CAD build for the part. Positions are in the model's coordinates, mm. A direction names the side the tool comes from. Coordinates: 2 decimals unless noted, no trailing zeros. Order: outer loops, then holes, each group sorted by start corner. A loop starts at its lowest first (then second) coordinate and runs counter-clockwise, first axis right, second up.
from build123d import *

# Parameters (mm, degrees)
SKETCH_R     = 4.1
SKETCH_R_2   = 1.6
SKETCH_W     = 24
SKETCH_H     = 2.341385
PAD_DEPTH    = 10
SKETCH001_W  = 16
SKETCH001_H  = 5
POCKET_DEPTH = 37
FILLET_R     = 5
FILLET001_R  = 1


with BuildPart() as part:
    # Sketch → Pad (new body)
    with BuildSketch(Plane(origin=(0, -80, 0), x_dir=(-1, 0, 0), z_dir=(0, 0, -1))):
        Polygon((0, 0), (-20, 0), (-20, 25), (-57, 33), (-57, 41), (3, 41), (3, 48), (14, 48), (14, 38), (12, 38), (12, 15), (34, 15), (34, 17), (44, 17), (44, 6), (0, 6), align=None)
        with Locations((-10, 11.430889)):
            Circle(SKETCH_R, mode=Mode.SUBTRACT)
        with Locations((-10, 31.430889)):
            Circle(SKETCH_R, mode=Mode.SUBTRACT)
        with Locations((9, 43.5)):
            Circle(SKETCH_R_2, mode=Mode.SUBTRACT)
        with Locations((9, 12.5)):
            Circle(SKETCH_R_2, mode=Mode.SUBTRACT)
        with Locations((40, 12.5)):
            Circle(SKETCH_R_2, mode=Mode.SUBTRACT)
        with Locations((-42, 36.829307)):
            Rectangle(SKETCH_W, SKETCH_H, mode=Mode.SUBTRACT)
    extrude(amount=PAD_DEPTH)

    # Sketch001 → Pocket (cut)
    with BuildSketch(Plane(origin=(57, -80, 0), x_dir=(0, -1, 0), z_dir=(1, 0, 0))):
        with Locations((-33, 2.5)):
            Rectangle(SKETCH001_W, SKETCH001_H)
    extrude(amount=-POCKET_DEPTH, mode=Mode.SUBTRACT)

    # Fillet
    fillet_edges = [part.edges().sort_by_distance(p)[0] for p in [
        (-44, -74, -5),
        (-44, -63, -5),
        (-14, -32, -5),
        (-3, -32, -5),
    ]]
    fillet(fillet_edges, radius=FILLET_R)

    # Fillet001
    fillet001_edges = [part.edges().sort_by_distance(p)[0] for p in [
        (-34, -63, -5),
        (-14, -42, -5),
    ]]
    fillet(fillet001_edges, radius=FILLET001_R)


solid = part.part
1) Slice it at B-B (x = -40). List the corners of the cut face in (y, z), plus the area to 3 significant figures.
2) Slice it at A-A (x = 10). List the corners of the cut face in (y, z), plus the area to 3 significant figures.
3) Drill centre lines: probe 1 along Y at (x, z) = (10, -6); probe 2 along Y at (x, z) = (-9, -7.25); probe 3 along X at (y, z) = (-66.5, -1.25). Where is each one in solid material? Low to high.
4) Pin check, flat tips, straight feed: P1, Ø4.5, axis at y = -38.5, z = -6, coming from the -X side; P2, Ø5, axis at x = 44, y = -45.5, coming from the +Z side; P3, Ø1.5, axis at y = -44.5, z = -8, coming from the -X side. Stop position of each tip, or through.
5) Slice it at D-D (z = -8.25). Give the number of separate pieces and of enclosed holes in the cut face, plus the area to 3 significant figures.
6) Two-plate mould, pull along X, no slides. Class faces 1 (the cylindrical face through (-13, -34, -5)), 2 (the flat face through (38.241, -51.056, -7.465)), 3 (the cylindrical face through (-8.792, -65.914, -4.93)), 4 (the flat face through (-20, -74, -5)): released by +X, released by -X, zero draft, split by the parting line, or undercut.
7) Slice it at C-C (z = -1). List the corners of the cut face in (x, y), plus the area to 3 significant figures.
8) Which spindle directions (+Z, -Z, +X, -X, +Y, -Y) get a long thin tool onto all of the face, cutting with end or side? Do faces 5 (the flat face through (20, -64, -5)), 6 (the flat face through (42, -44.341, -7)), 7 (the flat face through (-14, -39, -5)), 8 (the flat face through (21, -39, -6)). Say none if no direction does.
Worked out:
1. outline: (-73.9, -10) - (-69.1, -10) - (-69.1, 0) - (-73.9, 0) - close; (-65.9, -10) - (-63.1, -10) - (-63.1, 0) - (-65.9, 0) - close
1. area: 76.0 mm2
2. outline: (-80, -10) - (-72.67, -10) - (-72.67, 0) - (-80, 0) - close; (-64.47, -10) - (-52.67, -10) - (-52.67, 0) - (-64.47, 0) - close; (-44.47, -10) - (-39, -10) - (-39, 0) - (-44.47, 0) - close
2. area: 246 mm2
3. probe 1: y = -80 to -72.67, -64.47 to -52.67, -44.47 to -39
3. probe 2: y = -74 to -69.1, -65.9 to -38.1, -34.9 to -32
3. probe 3: x = -43.77 to -41.25, -38.75 to -10.25, -7.75 to 6.46, 13.54 to 20
4. P1: stops at x = -14
4. P2: stops at z = -5
4. P3: stops at x = -12
5. separate pieces: 1
5. enclosed holes: 6
5. area: 1,870 mm2
6. face 1: released by -X
6. face 2: released by +X
6. face 3: undercut
6. face 4: zero draft
7. outline: (-44, -69) arc R5 ccw to (-39, -74) - (0, -74) - (0, -80) - (20, -80) - (20, -39) - (-3, -39) - (-3, -37) arc R5 ccw to (-8, -32) - (-9, -32) arc R5 ccw to (-14, -37) - (-14, -41) arc R1 ccw to (-13, -42) - (-12, -42) - (-12, -65) - (-34, -65) - (-34, -64) arc R1 ccw to (-35, -63) - (-39, -63) arc R5 ccw to (-44, -68) - close; hole circle Ø3.2 at (-40, -67.5); hole circle Ø3.2 at (-9, -67.5); hole circle Ø3.2 at (-9, -36.5); hole circle Ø8.2 at (10, -68.57); hole circle Ø8.2 at (10, -48.57)
7. area: 1,480 mm2
8. face 5: +Z, +X, -Y
8. face 6: +Z, -Z
8. face 7: +Z, -Z, -X, +Y
8. face 8: +Z, -Z, +X, +Y
